Geometry: final body of the model. Coordinates: model frame, mm. Face numbers are marked on the shaded views. A direction names the side the tool comes from. Give positions to 0.01 mm unless a question says otherwise; leave off trailing zeros. Write each loop counter-clockwise with the first axis right and the second up, starting at its lowest first coordinate (ties: lowest second). Pieces come first, ordered by that corner, then holes. Notation, with made-up numbers: (51, 43) - (92, 43) arc R18 cw to (92, 56) - close; hole circle Ø5 at (31.25, -34). An arc over 180 degrees is marked (long way). Return JSON: item names as keys, results as strings.
from build123d import *

# Parameters (mm, degrees)
SKETCH1_W           = 24
SKETCH1_H           = 19
SKETCH1_R           = 1.65
BOSS_EXTRUDE1_DEPTH = 10
SKETCH2_R           = 3
CUT_EXTRUDE1_DEPTH  = 5.5
SKETCH4_W           = 24
SKETCH4_H           = 7
BOSS_EXTRUDE2_DEPTH = 8
SKETCH6_W           = 24
SKETCH6_H           = 10
BOSS_EXTRUDE3_DEPTH = 10
SKETCH7_R           = 1.65
CUT_EXTRUDE2_DEPTH  = 28
CUT_EXTRUDE3_DEPTH  = 2.2


with BuildPart() as part:
    # Sketch1 → Boss-Extrude1 (new body)
    with BuildSketch(Plane.XY):
        with Locations((-12, 37.5)):
            Rectangle(SKETCH1_W, SKETCH1_H)
        with Locations((-19.35, 37.5)):
            Circle(SKETCH1_R, mode=Mode.SUBTRACT)
        with Locations((-4.65, 37.5)):
            Circle(SKETCH1_R, mode=Mode.SUBTRACT)
    extrude(amount=BOSS_EXTRUDE1_DEPTH)

    # Sketch2 → Cut-Extrude1 (cut)
    with BuildSketch(Plane.XY.offset(10)):
        with Locations((-4.65, 37.5)):
            Circle(SKETCH2_R)
        with Locations((-19.35, 37.5)):
            Circle(SKETCH2_R)
    extrude(amount=-CUT_EXTRUDE1_DEPTH, mode=Mode.SUBTRACT)

    # Sketch4 → Boss-Extrude2 (add)
    with BuildSketch(Plane(origin=(0, 47, 0), x_dir=(1, 0, 0), z_dir=(0, 1, 0))):
        with Locations((-12, -6.5)):
            Rectangle(SKETCH4_W, SKETCH4_H)
    extrude(amount=BOSS_EXTRUDE2_DEPTH)

    # Sketch6 → Boss-Extrude3 (add)
    with BuildSketch(Plane.XY.offset(10)):
        with Locations((-12, 50)):
            Rectangle(SKETCH6_W, SKETCH6_H)
    extrude(amount=BOSS_EXTRUDE3_DEPTH)

    # Sketch7 → Cut-Extrude2 (cut, through all)
    with BuildSketch(Plane(origin=(0, 55, 0), x_dir=(1, 0, 0), z_dir=(0, 1, 0))):
        with Locations((-5.65, -14.829504021)):
            Circle(SKETCH7_R)
        with Locations((-18.35, -14.829504021)):
            Circle(SKETCH7_R)
    extrude(amount=-CUT_EXTRUDE2_DEPTH, mode=Mode.SUBTRACT)

    # Sketch8 → Cut-Extrude3 (cut)
    with BuildSketch(Plane.XZ.offset(-45)):
        Polygon((-2.359103466, 14.829504021), (-4.004551733, 17.679504021), (-7.295448267, 17.679504021), (-8.940896534, 14.829504021), (-7.295448267, 11.979504021), (-4.004551733, 11.979504021), align=None)
        Polygon((-15.059103466, 14.829504021), (-16.704551733, 17.679504021), (-19.995448267, 17.679504021), (-21.640896534, 14.829504021), (-19.995448267, 11.979504021), (-16.704551733, 11.979504021), align=None)
    extrude(amount=-CUT_EXTRUDE3_DEPTH, mode=Mode.SUBTRACT)


solid = part.part
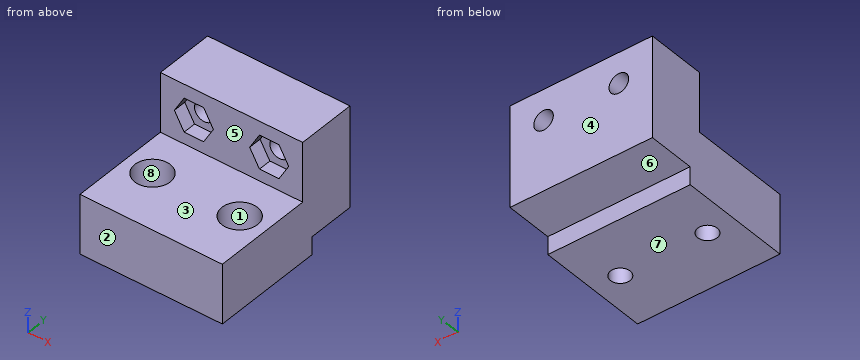
Q1. Section query B-B, the plane z = 7. Return the cut outline in (x, y).
Answer key:
{"outline": "(-24, 28) - (0, 28) - (0, 55) - (-24, 55) - close; hole circle Ø6 at (-19.35, 37.5); hole circle Ø6 at (-4.65, 37.5)"}
Q2. Material intervals for probe 1 along X at (y, z) = (47.5, 15); probe 2 along X at (y, z) = (37.5, 1.75); probe 3 along Y at (x, z) = (-19.35, 1.6), sorted ascending. Write a range as [from, to].
Answer key:
{"probe 1": "x = [-24, -19.99], [-16.71, -7.29], [-4.01, 0]", "probe 2": "x = [-24, -21], [-17.7, -6.3], [-3, 0]", "probe 3": "y = [28, 35.85], [39.15, 47]"}
Q3. Pin query (flat end, axial travel): P1, Ø6.5, axis at x = -4.5, z = 14, coming from the -Y side; P2, Ø2, axis at x = -15, y = 31, coming from the +Z side; P3, Ø4.5, axis at x = -5.65, z = 14.83, coming from the -Y side. Return the tip coordinate at first contact, or that it passes through.
Answer key:
{"P1": "stops at y = 45", "P2": "stops at z = 10", "P3": "stops at y = 47.2"}
Q4. Section query D-D, the plane y = 38. Return the cut outline in (x, z), plus the area to 3 significant figures.
Answer key:
{"outline": "(-24, 0) - (-20.92, 0) - (-20.92, 4.5) - (-22.31, 4.5) - (-22.31, 10) - (-24, 10) - close; (-17.78, 0) - (-6.22, 0) - (-6.22, 4.5) - (-7.61, 4.5) - (-7.61, 10) - (-16.39, 10) - (-16.39, 4.5) - (-17.78, 4.5) - close; (-3.08, 0) - (0, 0) - (0, 10) - (-1.69, 10) - (-1.69, 4.5) - (-3.08, 4.5) - close", "area": "147 mm^2"}
Q5. Set-up query: the marked faces 4, 5, 6, 7 and 8. Return all of +Z, -Z, +X, -X, +Y, -Y with unobstructed straight access to the full face (end or side cutting, diameter ignored); none if empty.
Answer key:
{"face 4": "+Z, -Z, +X, -X, +Y", "face 5": "+Z, +X, -X, -Y", "face 6": "-Z, +X, -X, +Y", "face 7": "-Z, +X, -X, +Y, -Y", "face 8": "+Z"}
Q6. Section query A-A, the plane y = 45.75. Return the cut outline in (x, z), plus the area to 3 significant figures.
Answer key:
{"outline": "(-24, 0) - (0, 0) - (0, 20) - (-24, 20) - close; hole (-21.64, 14.83) - (-20, 11.98) - (-16.7, 11.98) - (-15.06, 14.83) - (-16.7, 17.68) - (-20, 17.68) - close; hole (-8.94, 14.83) - (-7.3, 11.98) - (-4, 11.98) - (-2.36, 14.83) - (-4, 17.68) - (-7.3, 17.68) - close", "area": "424 mm^2"}
Q7. Mould query, pull axis Y, two halves, no side actions, for the marked faces 1, 2 and 3. Classes: pulls with the +Y half, pulls with the -Y half, needs draft (parallel to the pull), parting line crosses it, or undercut.
Answer key:
{"face 1": "undercut", "face 2": "pulls with the -Y half", "face 3": "needs draft"}
Q8. Section query C-C, the plane x = -19.5. Return the cut outline in (y, z), plus the area to 3 significant figures.
Answer key:
{"outline": "(28, 0) - (35.86, 0) - (35.86, 4.5) - (34.5, 4.5) - (34.5, 10) - (28, 10) - close; (39.14, 0) - (47, 0) - (47, 3) - (55, 3) - (55, 13.65) - (47.2, 13.65) - (47.2, 11.98) - (45, 11.98) - (45, 10) - (40.5, 10) - (40.5, 4.5) - (39.14, 4.5) - close; (45, 17.68) - (47.2, 17.68) - (47.2, 16.01) - (55, 16.01) - (55, 20) - (45, 20) - close", "area": "267 mm^2"}
